from build123d import *

# Parameters (mm, degrees)
SKETCH1_R                  = 6.4
BOSS_EXTRUDE1_DEPTH        = 165
F_10_24_TAPPED_HOLE1_D     = 3.7973
F_10_24_TAPPED_HOLE1_DEPTH = 12.83
F_10_24_TAPPED_HOLE1_TIP   = 1.140824014
F_10_24_TAPPED_HOLE2_D     = 3.7973
F_10_24_TAPPED_HOLE2_DEPTH = 12.83
F_10_24_TAPPED_HOLE2_TIP   = 1.140824014


with BuildPart() as part:
    # Sketch1 → Boss-Extrude1 (new body)
    with BuildSketch(Plane.XY):
        Circle(SKETCH1_R)
    extrude(amount=BOSS_EXTRUDE1_DEPTH)

    # #10-24 Tapped Hole1
    with Locations(Plane(origin=(0, 0, 0), x_dir=(-1, 0, 0), z_dir=(0, 0, -1))):
        with Locations((0, 0)):
            Hole(F_10_24_TAPPED_HOLE1_D / 2, depth=F_10_24_TAPPED_HOLE1_DEPTH)
            with Locations((0, 0, -(F_10_24_TAPPED_HOLE1_DEPTH + F_10_24_TAPPED_HOLE1_TIP / 2))):  # 118° drill point
                Cone(0, F_10_24_TAPPED_HOLE1_D / 2, F_10_24_TAPPED_HOLE1_TIP, mode=Mode.SUBTRACT)

    # #10-24 Tapped Hole2
    with Locations(Plane.XY.offset(165)):
        with Locations((0, 0)):
            Hole(F_10_24_TAPPED_HOLE2_D / 2, depth=F_10_24_TAPPED_HOLE2_DEPTH)
            with Locations((0, 0, -(F_10_24_TAPPED_HOLE2_DEPTH + F_10_24_TAPPED_HOLE2_TIP / 2))):  # 118° drill point
                Cone(0, F_10_24_TAPPED_HOLE2_D / 2, F_10_24_TAPPED_HOLE2_TIP, mode=Mode.SUBTRACT)


solid = part.part
Geometry: final body of the model. Coordinates: model frame, mm. A direction names the side the tool comes from. Give positions to 0.01 mm unless a question says otherwise; leave off trailing zeros. Order: outer loops, then holes, each group sorted by start corner. A loop starts at its lowest first (then second) coordinate and runs counter-clockwise, first axis right, second up. Notation, with made-up numbers: (-38.75, 28.25) - (-24.75, 28.25) arc R24 cw to (-24.75, 67.25) - close; hole circle Ø6 at (-27, -27). An arc over 180 degrees is marked (long way). Use CSV: the item, a comma, the result in double quotes.
1. Section query A-A (z = 56.5). Output: boundary loops of the cut face in (x, y).
Answers below:
outline,"circle Ø12.8 at (0, 0)"
2. Section query C-C (y = 4.5). Output: boundary loops of the cut face in (x, z), plus the area to 3 significant figures.
Answers below:
outline,"(-4.55, 0) - (4.55, 0) - (4.55, 165) - (-4.55, 165) - close"
area,"1,500 mm2"
3. Material intervals for line 1 along Y through (x, z) = (0, 155.5); line 2 along X through (y, z) = (-3.25, 39); line 3 along Y through (x, z) = (3.5, 26), sorted ascending. Write a range as from..to.
Answers below:
line 1,"-6.4..-1.9, 1.9..6.4"
line 2,"-5.51..5.51"
line 3,"-5.36..5.36"
4. Mould query, pull axis Y, two halves, no side actions, for faces 4 (the face through (-5.08, -3.89, 81.34)), 5 (the face through (1, 2, 165)), 6 (the face through (0.315, 0.099, 151.227)). Classes: +Y half, -Y half, draft (parallel to the pull), parting line (faces both ways), or undercut.
Answers below:
face 4,"parting line"
face 5,"draft"
face 6,"undercut"
5. Section query B-B (x = 3.75). Output: boundary loops of the cut face in (y, z).
Answers below:
outline,"(-5.19, 0) - (5.19, 0) - (5.19, 165) - (-5.19, 165) - close"
6. Access query for faces 1 (the face through (1, 2, 0)), 2 (the face through (1.8, 0.6, 6.5)), 3 (the face through (-1.8, 0.6, 158.5)). Directions: +Z, -Z, +X, -X, +Y, -Y. A direction counts if a zero-diameter tool reaches every point of the face in a straight line with its end or side. Return the directions, or none.
Answers below:
face 1,"-Z, +X, -X, +Y, -Y"
face 2,"-Z"
face 3,"+Z"
7. Contact query for flat-ended pins moving along their axis: pin 1 (4 mm diameter, centred on y = -2.5, z = 105, fed in from -X); pin 2 (2 mm diameter, centred on x = 0.5, y = -0.5, fed in from +Z); pin 3 (1 mm diameter, centred on x = -1.5, z = 61.5, fed in from -Y). Output: stop coordinate, or through.
Answers below:
pin 1,"x = -6.38"
pin 2,"z = 152.05"
pin 3,"y = -6.32"
